Autodesk Inventor part; units mm, degrees
ref_plane "YZ Plane" through (0, 0, 0) normal (1, 0, 0) x (0, 1, 0)
ref_plane "XZ Plane" through (0, 0, 0) normal (0, 1, 0) x (-1, 0, 0)
ref_plane "XY Plane" through (0, 0, 0) normal (0, 0, 1) x (1, 0, 0)
sketch "Sketch_1" plane through (0, 0, 0) normal (0, 0, 1) x (1, 0, 0)
  line L0 (5, 0) -> (0, 0)
  line L1 (0, 10.05) -> (5, 10.05)
  line L2 (5, 10.05) -> (5, 12.85)
  arc A0 (5, 12.85) -> (4.85, 13) centre (4.85, 12.85) ccw
  line L3 (4.85, 13) -> (0.15, 13)
  arc A1 (0.15, 13) -> (0, 12.85) centre (0.15, 12.85) ccw
  line L4 (0, 12.85) -> (0, 10.05)
revolve "Revolution1" add sketch "Sketch_1" angle 360 about axis through (5, 0, 0) along (1, 0, 0)
sketch "Sketch_4" plane through (0, 0, 0) normal (0, 0, 1) x (1, 0, 0)
  line L0 (3.5, 0) -> (1.5, 0)
  line L1 (1.0858, 9.8) -> (2.5, 8.3858)
  line L2 (2.5, 8.3858) -> (3.9142, 9.8)
  line L3 (3.9142, 9.8) -> (2.5, 11.2142)
  line L4 (2.5, 11.2142) -> (1.0858, 9.8)
revolve "Revolution2" cut sketch "Sketch_4" angle 360 about axis through (3.5, 0, 0) along (1, 0, 0)
properties part number "CRBT155A_PART2" material "ステンレス鋼"
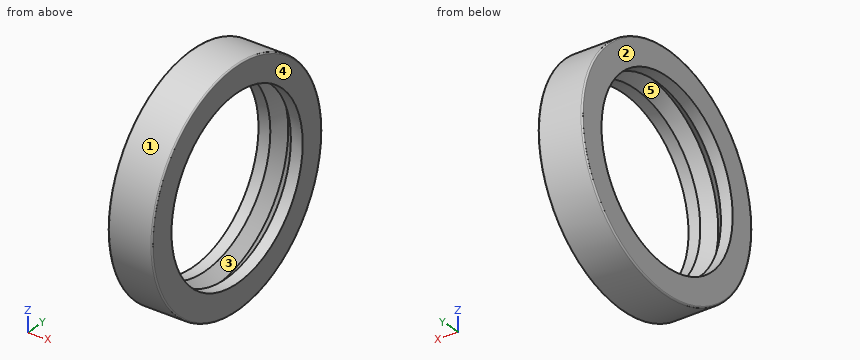
Build history of the part. All positions in model axes, mm. Face numbers are marked on the shaded views. A direction names the side the tool comes from. Give positions to 0.01 mm unless a question says otherwise; leave off trailing zeros. Loops run counter-clockwise (first coordinate to the right, second up) from the corner with the lowest first, then second, coordinate; pieces in that order, holes last. Notation, with made-up numbers: (56.25, 82.5) -> (100.25, 82.5) arc R33 ccw to (100.25, 111.5) -> close; hole circle Ø3 at (42.5, 23). An arc over 180 degrees is marked (long way). One line per question, with ' | ' between items. Start each with the question number.
1) Two-plate mould, pull along Z, no slides. Class the marked faces 1, 2 and 3: released by +Z, released by -Z, zero draft, split by the parting line, or undercut.
2) Probe L1, parallel to Z at x = 0.8, y = 0; L2, parallel to Y at x = 4.8, z = -6.25; L3, parallel to Z at x = 1.5, y = -7.5. List the from-to ranges inside material, lowest first.
3) Cut at C-C (x = 4). Give the cut face in (y, z).
4) Cut at A-A (z = 0). Give the cut face in (x, y), plus the area to 3 significant figures.
5) Pin check, flat tip, straight feed: pin 1 (3 mm diameter, centred on x = 3.5, z = 9, fed in from -Y). Stop position of the tip, or through.
6) 3-axis set-ups, long thin cutter, end or side, ignore diameter. For the marked faces 4 and 5: which of +Z, -Z, +X, -X, +Y, -Y reach the whole face in a straight line?
Return value:
1) face 1: split by the parting line | face 2: zero draft | face 3: undercut
2) L1: -13 to -10.05, 10.05 to 13 | L2: -11.4 to -7.87, 7.87 to 11.4 | L3: -10.62 to -6.93, 6.93 to 10.62
3) outline: circle Ø26 at (0, 0); hole circle Ø20.1 at (0, 0)
4) outline: (0, -12.85) arc R0.15 ccw to (0.15, -13) -> (4.85, -13) arc R0.15 ccw to (5, -12.85) -> (5, -10.05) -> (3.66, -10.05) -> (2.5, -11.21) -> (1.34, -10.05) -> (0, -10.05) -> close; (0, 10.05) -> (1.34, 10.05) -> (2.5, 11.21) -> (3.66, 10.05) -> (5, 10.05) -> (5, 12.85) arc R0.15 ccw to (4.85, 13) -> (0.15, 13) arc R0.15 ccw to (0, 12.85) -> close | area: 26.8 mm^2
5) pin 1: y = -10.62
6) face 4: +Z, -Z, +X, +Y, -Y | face 5: none
